from build123d import *

# Parameters (mm, degrees)
BOSS_EXTRUDE2_DEPTH = 24
SKETCH2_R           = 25.5
BOSS_EXTRUDE3_DEPTH = 5
SKETCH3_W           = 44
SKETCH3_H           = 28
BOSS_EXTRUDE4_DEPTH = 132
FILLET2_R           = 14
FILLET5_R           = 14
SKETCH4_R           = 7.25
BOSS_EXTRUDE5_DEPTH = 20


with BuildPart() as part:
    # Sketch1 → Boss-Extrude2 (new body)
    with BuildSketch(Plane(origin=(0, 0, 0), x_dir=(1, 0, 0), z_dir=(0, 1, 0))):
        with BuildLine():
            Line((-114, 26), (0, 26))
            ThreePointArc((0, 26), (26, 0), (0, -26))
            Line((0, -26), (-114, -26))
            Line((-114, -26), (-114, 26))
        make_face()
    extrude(amount=BOSS_EXTRUDE2_DEPTH)

    # Sketch2 → Boss-Extrude3 (add)
    with BuildSketch(Plane.XZ):
        with Locations(Location((0, 0, 0), (0, 0, 90))):
            Circle(SKETCH2_R)
    extrude(amount=BOSS_EXTRUDE3_DEPTH)

    # Sketch3 → Boss-Extrude4 (add)
    with BuildSketch(Plane(origin=(0, 0, 0), x_dir=(1, 0, 0), z_dir=(0, 1, 0))):
        with Locations((-114, 0)):
            Rectangle(SKETCH3_W, SKETCH3_H)
    extrude(amount=BOSS_EXTRUDE4_DEPTH)

    # Fillet2
    fillet2_edges = [part.edges().sort_by_distance(p)[0] for p in [
        (-114, 132, 14),
    ]]
    fillet(fillet2_edges, radius=FILLET2_R)

    # Fillet5
    fillet5_edges = [part.edges().sort_by_distance(p)[0] for p in [
        (-114, 132, -14),
    ]]
    fillet(fillet5_edges, radius=FILLET5_R - 0.0001)  # a hair under: the kernel refuses the full size

    # Sketch4 → Boss-Extrude5 (add)
    with BuildSketch(Plane(origin=(-92, 0, 0), x_dir=(0, 0, -1), z_dir=(1, 0, 0))):
        with Locations(Location((0, 118, 0), (0, 0, 180))):
            Circle(SKETCH4_R)
    extrude(amount=BOSS_EXTRUDE5_DEPTH)


solid = part.part
Model file for the job. Use its own axes, mm. A direction names the side the tool comes from. Give positions to 0.01 mm unless a question says otherwise; leave off trailing zeros. Loops run counter-clockwise (first coordinate to the right, second up) from the corner with the lowest first, then second, coordinate; pieces in that order, holes last. Notation, with made-up numbers: (26, 86.5) -> (37, 86.5) arc R8 ccw to (37, 95.5) -> close; hole circle Ø10 at (-23, -1.5). An arc over 180 degrees is marked (long way). Use a Markdown table: item, result. Add a question column.
(1) Slice it at D-D on y = 45. List the corners of the cut face in (x, z).
(2) Mould opens along Y. For faces 4 (the cylindrical face through (-113.7, 127.8, 10)), 5 (the cylindrical face through (-82.14, 124.43, 3.35)), 6 (the flat face through (-114, 12, -20)) say: +Y half, -Y half, draft (parallel to the pull), parting line (faces both ways), or undercut.
(3) Wall check: line 1 along X through (y, z) = (110, -2.5); line 2 along Y through (x, z) = (-106, 23); line 3 along Z through (x, y) = (-93, 114). Give the ranges that are in metal, low to high.
(4) Tool access for faces 1 (the flat face through (-72, 118, 0)), 2 (the flat face through (-114, 12, 20)), 3 (the cylindrical face through (24.9, -2.5, -5.5)): list every direction of +Z, -Z, +X, -X, +Y, -Y with a clear straight run to the whole face (end or side of a thin tool).
(5) Drop flat-ended pins along their axis: pin 1 Ø4.5 at (y, z) = (118, -1.5) entering from +X; pin 2 Ø13 at (y, z) = (11, 21.5) entering from -X; pin 3 Ø3 at (x, z) = (-107.5, 4.5) entering from +Y. Give the stop position or say it passes through.
(6) Slice it at C-C on z = 16.5. List the corners of the cut face in (x, y).
(7) Slice it at A-A on x = -85. List the corners of the cut face in (y, z).
Filled sheet:
| question | item | result |
|---|---|---|
| 1 | outline | (-136, -14) -> (-92, -14) -> (-92, 14) -> (-136, 14) -> close |
| 2 | face 4 | +Y half |
| 2 | face 5 | undercut |
| 2 | face 6 | draft |
| 3 | line 1 | -136 to -92 |
| 3 | line 2 | 0 to 24 |
| 3 | line 3 | -14 to 14 |
| 4 | face 1 | +Z, -Z, +X, +Y |
| 4 | face 2 | +Z, -X, +Y, -Y |
| 4 | face 3 | -Y |
| 5 | pin 1 | x = -72 |
| 5 | pin 2 | x = -114 |
| 5 | pin 3 | y = 131.67 |
| 6 | outline | (-114, 0) -> (-19.44, 0) -> (-19.44, -5) -> (19.44, -5) -> (19.44, 0) -> (20.09, 0) -> (20.09, 24) -> (-114, 24) -> close |
| 7 | outline | (0, -26) -> (24, -26) -> (24, 26) -> (0, 26) -> close; circle Ø14.5 at (118, 0) |
